```python
from build123d import *

# Parameters (mm, degrees)
SKETCH_1_W          = 7.2
SKETCH_1_H          = 116
EXTRUDE_1_DEPTH     = 2.5
SHELL_1_T           = -0.2
CUT_EXTRUDE_1_DEPTH = 2.5


with BuildPart() as part:
    # 스케치1 → 보스-돌출1 (new body)
    with BuildSketch(Plane.XY):
        with Locations((3.6, 58)):
            Rectangle(SKETCH_1_W, SKETCH_1_H)
    extrude(amount=EXTRUDE_1_DEPTH)

    # 쉘1
    shell_1_openings = [part.faces().sort_by_distance(p)[0] for p in [
        (3.6, 58, 2.5),
    ]]
    offset(amount=SHELL_1_T, openings=shell_1_openings, kind=Kind.INTERSECTION)

    # 스케치2 → 컷-돌출1 (cut)
    with BuildSketch(Plane.XY.offset(0.2)):
        with BuildLine():
            Line((5.6, 108), (5.6, 8))
            ThreePointArc((5.6, 8), (3.6, 6), (1.6, 8))
            Line((1.6, 8), (1.6, 108))
            ThreePointArc((1.6, 108), (3.6, 110), (5.6, 108))
        make_face()
    extrude(amount=-CUT_EXTRUDE_1_DEPTH, mode=Mode.SUBTRACT)


solid = part.part
```
Geometry: final body of the model. Coordinates: model frame, mm. A direction names the side the tool comes from. Round coordinates to 2 decimals unless told otherwise and drop trailing zeros. Loops run counter-clockwise (first coordinate to the right, second up) from the corner with the lowest first, then second, coordinate; pieces in that order, holes last.
Item 1: Section C-C, the plane z = 1.2. Output: boundary loops of the cut face in (x, y).
Checked values:
outline: (0, 0) - (7.2, 0) - (7.2, 116) - (0, 116) - close; hole (0.2, 0.2) - (7, 0.2) - (7, 115.8) - (0.2, 115.8) - close
Item 2: Contact query for flat-ended pins moving along their axis: P1, Ø1, axis at x = 5.5, y = 99.5, coming from the +Z side; P2, Ø2, axis at x = 4.5, y = 79, coming from the +Z side. Output: stop coordinate, or through.
Checked values:
P1: stops at z = 0.2
P2: passes through
Item 3: Section B-B, the plane y = 81.5. Output: boundary loops of the cut face in (x, z).
Checked values:
outline: (0, 0) - (1.6, 0) - (1.6, 0.2) - (0.2, 0.2) - (0.2, 2.5) - (0, 2.5) - close; (5.6, 0) - (7.2, 0) - (7.2, 2.5) - (7, 2.5) - (7, 0.2) - (5.6, 0.2) - close
Item 4: Section A-A, the plane x = 3.6. Output: boundary loops of the cut face in (y, z).
Checked values:
outline: (0, 0) - (6, 0) - (6, 0.2) - (0.2, 0.2) - (0.2, 2.5) - (0, 2.5) - close; (110, 0) - (116, 0) - (116, 2.5) - (115.8, 2.5) - (115.8, 0.2) - (110, 0.2) - close
Item 5: Reachability of faces 1 (the flat face through (1, 59, 0.2)), 2 (the flat face through (0, 57, 1)) from +Z, -Z, +X, -X, +Y, -Y: full face, straight path, thin tool, end or side. Return the list, or none.
Checked values:
face 1: +Z
face 2: +Z, -Z, -X, +Y, -Y
Item 6: Mould query, pull axis Y, two halves, no side actions, for faces 3 (the flat face through (7, 57, 1)), 4 (the flat face through (4, 0, 1)), 5 (the flat face through (1, 59, 0)). Classes: released by +Y, released by -Y, zero draft, split by the parting line, or undercut.
Checked values:
face 3: undercut
face 4: released by -Y
face 5: zero draft
Item 7: Line query: L1, parallel to Y at x = 3.25, z = 1.7; L2, parallel to X at y = 31.5, z = 1.35; L3, parallel to Z at x = 6, y = 83. Output: solid intervals per line, ascending.
Checked values:
L1: y = 0 to 0.2, 115.8 to 116
L2: x = 0 to 0.2, 7 to 7.2
L3: z = 0 to 0.2
